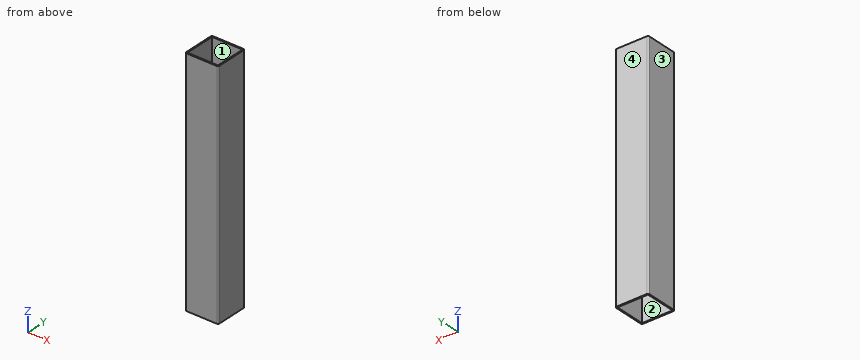
from build123d import *

# Parameters (mm, degrees)
CROQUIS1_W              = 23.4
CROQUIS1_H              = 23.4
SALIENTE_EXTRUIR1_DEPTH = 180


with BuildPart() as part:
    # Croquis1 → Saliente-Extruir1 (new body)
    with BuildSketch(Plane.XY):
        with BuildLine():
            Line((-11.7, -12.7), (11.7, -12.7))
            ThreePointArc((11.7, -12.7), (12.407106781, -12.407106781), (12.7, -11.7))
            Line((12.7, -11.7), (12.7, 11.7))
            ThreePointArc((12.7, 11.7), (12.407106781, 12.407106781), (11.7, 12.7))
            Line((11.7, 12.7), (-11.7, 12.7))
            ThreePointArc((-11.7, 12.7), (-12.407106781, 12.407106781), (-12.7, 11.7))
            Line((-12.7, 11.7), (-12.7, -11.7))
            ThreePointArc((-12.7, -11.7), (-12.407106781, -12.407106781), (-11.7, -12.7))
        make_face()
        Rectangle(CROQUIS1_W, CROQUIS1_H, mode=Mode.SUBTRACT)
    extrude(amount=-SALIENTE_EXTRUIR1_DEPTH)


solid = part.part
Here's how the part is built. I have some questions about the finished solid (model axes, mm). Face numbers are marked on the shaded views. Round coordinates to 2 decimals unless told otherwise and drop trailing zeros. Loops run counter-clockwise (first coordinate to the right, second up) from the corner with the lowest first, then second, coordinate; pieces in that order, holes last. Notation, with made-up numbers: (-37.75, -29.5) -> (5.25, -29.5) arc R13 cw to (5.25, -7.5) -> close; hole circle Ø4 at (26, 8). An arc over 180 degrees is marked (long way). Write each question's results on one line, items separated by ' | '.
(1) If we section it at A-A, the plane x = 6.75: List the corners of the cut face in (y, z) for me.
Worked answers:
outline: (-12.7, -180) -> (-11.7, -180) -> (-11.7, 0) -> (-12.7, 0) -> close; (11.7, -180) -> (12.7, -180) -> (12.7, 0) -> (11.7, 0) -> close
(2) If we section it at C-C, the plane z = -91.5: List the corners of the cut face in (x, y) for me, then the cut area to 3 significant figures.
Worked answers:
outline: (-12.7, -11.7) arc R1 ccw to (-11.7, -12.7) -> (11.7, -12.7) arc R1 ccw to (12.7, -11.7) -> (12.7, 11.7) arc R1 ccw to (11.7, 12.7) -> (-11.7, 12.7) arc R1 ccw to (-12.7, 11.7) -> close; hole (-11.7, -11.7) -> (11.7, -11.7) -> (11.7, 11.7) -> (-11.7, 11.7) -> close | area: 96.7 mm2
(3) We'd pull the mould along Y, two halves only. Please class the marked faces 1, 2, 3 and 4: released by +Y, released by -Y, zero draft, split by the parting line, or undercut.
Worked answers:
face 1: undercut | face 2: undercut | face 3: zero draft | face 4: released by +Y
(4) If I drill on L1, parallel to X at y = -7, z = -77, over which ranges is the centre line in solid material (lowest first)?
Worked answers:
L1: -12.7 to -11.7, 11.7 to 12.7
